The figure shows three views and two pictorial views of one solid part (mm, origin at its lowest corner). Answer the questions. A direction names the side the tool comes from. Round coordinates to 2 decimals unless told otherwise and drop trailing zeros. Loops run counter-clockwise (first coordinate to the right, second up) from the corner with the lowest first, then second, coordinate; pieces in that order, holes last. Notation, with made-up numbers: (-26, 87.25) -> (-14, 87.25) arc R24 cw to (-14, 121.25) -> close; hole circle Ø3 at (-30.5, 86). An arc over 180 degrees is marked (long way). Put each result on its own line as item: value.
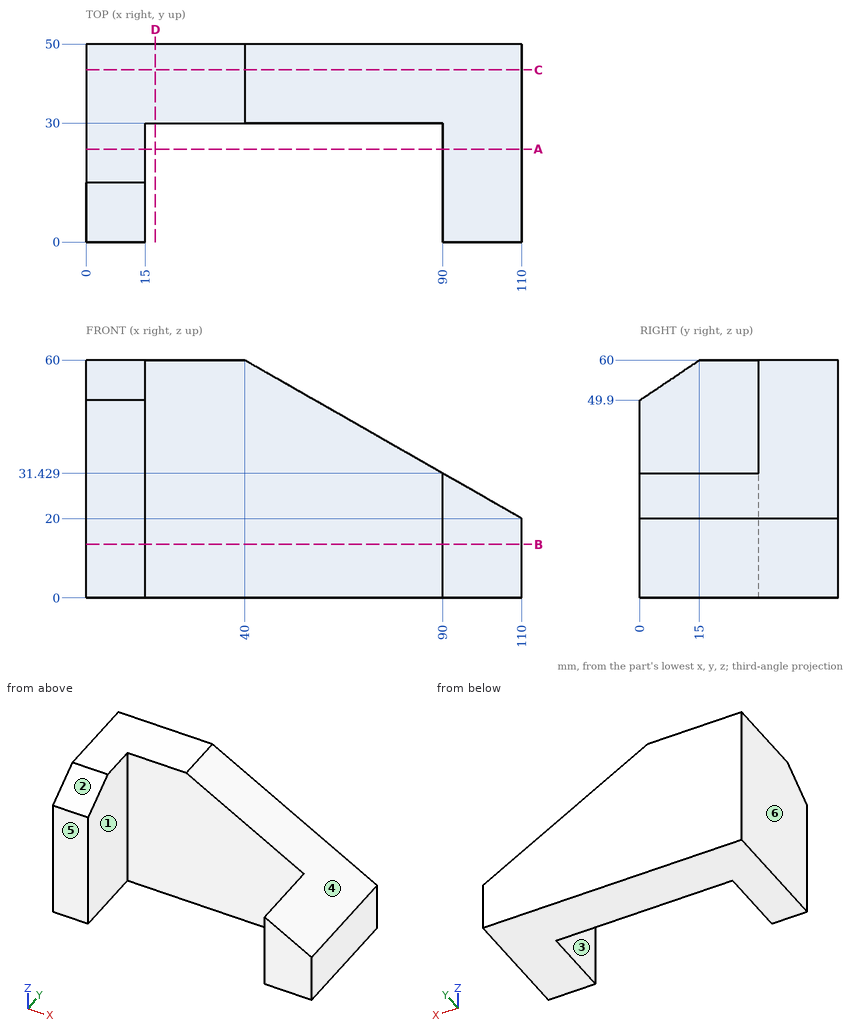
Item 1: The part is cut by section D-D (x = 17.5). Determine the outline of the cut face in (y, z).
Derived:
outline: (30, 0) -> (50, 0) -> (50, 60) -> (30, 60) -> close
Item 2: The part is cut by section B-B (z = 13.5). Determine the outline of the cut face in (x, y).
Derived:
outline: (0, 0) -> (15, 0) -> (15, 30) -> (90, 30) -> (90, 0) -> (110, 0) -> (110, 50) -> (0, 50) -> close
Item 3: Which of the six approach directions +Z, -Z, +X, -X, +Y, -Y give full straight-line access (tool end or side, diameter ignored) to the marked faces 1 and 2?
Derived:
face 1: +Z, -Z, -Y
face 2: +Z, +X, -X, -Y
Item 4: The part is cut by section A-A (y = 23.5). Determine the outline of the cut face in (x, z).
Derived:
outline: (0, 0) -> (15, 0) -> (15, 60) -> (0, 60) -> close; (90, 0) -> (110, 0) -> (110, 20) -> (90, 31.43) -> close
Item 5: Flat-ended cylindrical pins translate along their axes: pin 1 Ø12 at (x, z) = (84.5, 40) entering from -Y; pin 2 Ø15 at (y, z) = (10.5, 12) entering from -X; pin 3 Ø2 at (y, z) = (29, 26) entering from +X. Find the tip coordinate at first contact, or state that the pin passes through.
Derived:
pin 1: stops at y = 30
pin 2: stops at x = 0
pin 3: stops at x = 101.25
Item 6: The part is cut by section C-C (y = 43.5). Determine the outline of the cut face in (x, z).
Derived:
outline: (0, 0) -> (110, 0) -> (110, 20) -> (40, 60) -> (0, 60) -> close
Item 7: For a pull along X with two mould halves and no side action, classify the marked faces 3, 4, 5 and 6 as pulls with the +X half, pulls with the -X half, needs draft (parallel to the pull), parting line crosses it, or undercut.
Derived:
face 3: undercut
face 4: pulls with the +X half
face 5: needs draft
face 6: pulls with the -X half
Item 8: Find the intervals of material crossed by line 1 along Y through (x, z) = (79, 11); line 2 along X through (y, z) = (29, 37.5); line 3 along X through (y, z) = (22.5, 21), in increasing order.
Derived:
line 1: y = 30 to 50
line 2: x = 0 to 15
line 3: x = 0 to 15, 90 to 108.25
